Geometry: final body of the model. Coordinates: model frame, mm. Face numbers are marked on the shaded views. Coordinates: 2 decimals unless noted, no trailing zeros. Loops run counter-clockwise (first coordinate to the right, second up) from the corner with the lowest first, then second, coordinate; pieces in that order, holes last. Notation, with made-up numbers: (35.5, 56) - (86.5, 56) arc R33 ccw to (86.5, 94) - close; hole circle Ø6 at (-17, -24.5). An arc over 180 degrees is marked (long way). Return JSON: item names as keys, results as strings.
from build123d import *

# Parameters (mm, degrees)
BOSS_EXTRU_1_DEPTH = 1.7
ESQUISSE2_W        = 3
ESQUISSE2_H        = 4
BOSS_EXTRU_2_DEPTH = 7.5
ESQUISSE3_W        = 5
ESQUISSE3_H        = 32
BOSS_EXTRU_3_DEPTH = 2.85
CONG_1_R           = 5
ESQUISSE4_W        = 4
ESQUISSE4_H        = 2
BOSS_EXTRU_4_DEPTH = 0.65


with BuildPart() as part:
    # Esquisse1 → Boss.-Extru.1 (new body)
    with BuildSketch(Plane(origin=(0, 0, 0), x_dir=(1, 0, 0), z_dir=(0, 1, 0))):
        Polygon((-12, 4), (-9, 4), (-9, 2), (9, 2), (9, 4), (12, 4), (12, 0), (-12, 0), align=None)
    extrude(amount=BOSS_EXTRU_1_DEPTH)

    # Esquisse2 → Boss.-Extru.2 (add)
    with BuildSketch(Plane(origin=(0, 1.7, 0), x_dir=(1, 0, 0), z_dir=(0, 1, 0))):
        with Locations((-10.5, 2)):
            Rectangle(ESQUISSE2_W, ESQUISSE2_H)
        with Locations((10.5, 2)):
            Rectangle(ESQUISSE2_W, ESQUISSE2_H)
    extrude(amount=BOSS_EXTRU_2_DEPTH)

    # Esquisse3 → Boss.-Extru.3 (add)
    with BuildSketch(Plane(origin=(0, 9.2, 0), x_dir=(1, 0, 0), z_dir=(0, 1, 0))):
        with Locations((-9.5, 16)):
            Rectangle(ESQUISSE3_W, ESQUISSE3_H)
        with Locations((9.5, 16)):
            Rectangle(ESQUISSE3_W, ESQUISSE3_H)
    extrude(amount=-BOSS_EXTRU_3_DEPTH)

    # Congé1
    cong_1_edges = [part.edges().sort_by_distance(p)[0] for p in [
        (9.5, 9.2, 0),
        (-9.5, 9.2, 0),
    ]]
    fillet(cong_1_edges, radius=CONG_1_R)

    # Esquisse4 → Boss.-Extru.4 (add)
    with BuildSketch(Plane(origin=(0, 1.7, 0), x_dir=(1, 0, 0), z_dir=(0, 1, 0))):
        with Locations((-7, 1)):
            Rectangle(ESQUISSE4_W, ESQUISSE4_H)
        with Locations((7, 1)):
            Rectangle(ESQUISSE4_W, ESQUISSE4_H)
    extrude(amount=BOSS_EXTRU_4_DEPTH)


solid = part.part
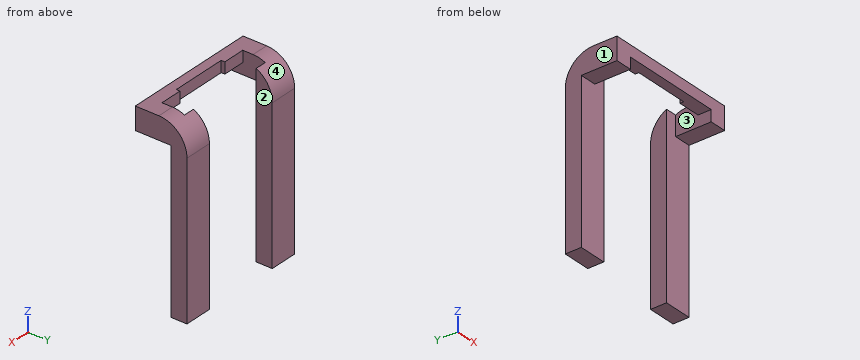
Item 1: Section query C-C, the plane x = 10.25. Return loops of the section in (y, z), and give its area (3 significant figures).
Worked out:
{"outline": "(0, -4) - (6.35, -4) - (6.35, -32) - (9.2, -32) - (9.2, -5) arc R5 ccw to (4.2, 0) - (0, 0) - close", "area": "111 mm^2"}
Item 2: First-contact query: pin 1 Ø1.5 at (x, z) = (-10, -21) entering from -Y; pin 2 Ø1.5 at (x, y) = (10.5, 4) entering from -Z; pin 3 Ø2 at (x, z) = (0.5, -0.5) entering from +Y. Flat tips, straight axial feed; report the tip coordinate or a pass-through.
Worked out:
{"pin 1": "y = 6.35", "pin 2": "z = -4", "pin 3": "y = 1.7"}
Item 3: Mould query, pull axis X, two halves, no side actions, for the marked faces 1, 2, 3 and 4. Classes: +X half, -X half, draft (parallel to the pull), parting line (faces both ways), or undercut.
Worked out:
{"face 1": "-X half", "face 2": "undercut", "face 3": "undercut", "face 4": "draft"}
Item 4: Section query B-B, the plane y = 2.75. Return loops of the section in (x, z).
Worked out:
{"outline": "(-12, -4) - (-9, -4) - (-9, 0) - (-12, 0) - close; (9, -4) - (12, -4) - (12, 0) - (9, 0) - close"}
Item 5: Section query A-A, the plane z = -7.5. Return loops of the section in (x, y), and give its area (3 significant figures).
Worked out:
{"outline": "(-12, 6.35) - (-7, 6.35) - (-7, 9.2) - (-12, 9.2) - close; (7, 6.35) - (12, 6.35) - (12, 9.2) - (7, 9.2) - close", "area": "28.5 mm^2"}
Item 6: Section query D-D, the plane x = 6. Return loops of the section in (y, z).
Worked out:
{"outline": "(0, -2) - (2.35, -2) - (2.35, 0) - (0, 0) - close"}
Item 7: Ray query, probe 1 along X at (y, z) = (7.75, -15.5); probe 2 along Z at (x, y) = (10.75, 1.25); probe 3 along Z at (x, y) = (-6, 0.5). Return the intervals inside material, ascending. Write a range as from..to.
Worked out:
{"probe 1": "-12..-7, 7..12", "probe 2": "-4..0", "probe 3": "-2..0"}
